Can you work these out from the drawing? Everything is in mm from the part's minimum corner. A direction names the side the tool comes from. Give positions to 0.01 mm unless a question says otherwise; leave off trailing zeros. Order: outer loops, then holes, each group sorted by start corner. A loop starts at its lowest first (then second) coordinate and runs counter-clockwise, first axis right, second up. Notation, with made-up numbers: (24.5, 53) -> (79.5, 53) arc R32 cw to (79.5, 83) -> close; hole circle Ø6 at (-30.75, -40). An arc over 180 degrees is marked (long way). One line per item, written item: value.
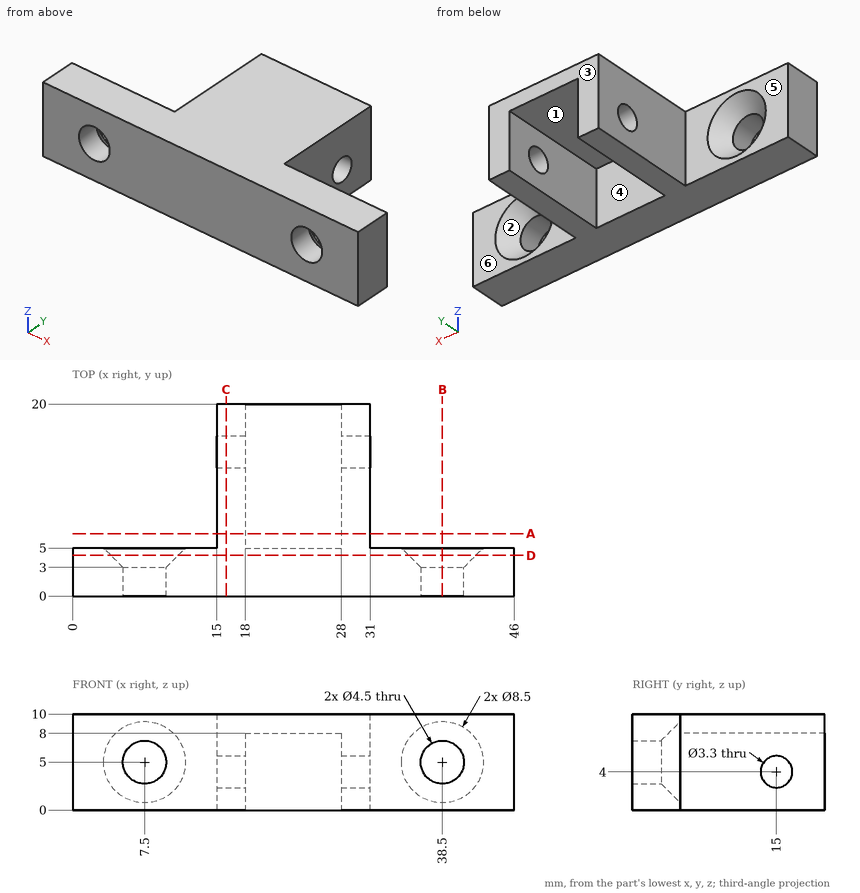
1) Suppose I cut it at C-C, the plane x = 16. Write out the boundary of the cut face in (y, z).
Answer below:
outline: (0, 0) -> (20, 0) -> (20, 10) -> (0, 10) -> close; hole circle Ø3.3 at (15, 4)
2) We'd pull the mould along Z, two halves only. Please class the marked faces 1, 2 and 3: +Z half, -Z half, draft (parallel to the pull), parting line (faces both ways), or undercut.
Answer below:
face 1: -Z half
face 2: undercut
face 3: draft
3) Suppose I cut it at B-B, the plane x = 38.5. Write out the boundary of the cut face in (y, z), then the cut area to 3 significant figures.
Answer below:
outline: (0, 0) -> (5, 0) -> (5, 0.75) -> (3, 2.75) -> (0, 2.75) -> close; (0, 7.25) -> (3, 7.25) -> (5, 9.25) -> (5, 10) -> (0, 10) -> close
area: 23.5 mm2
4) Suppose I cut it at D-D, the plane y = 4.25. Write out the boundary of the cut face in (x, z), then the cut area to 3 significant figures.
Answer below:
outline: (0, 0) -> (46, 0) -> (46, 10) -> (0, 10) -> close; hole circle Ø7 at (7.5, 5); hole circle Ø7 at (38.5, 5)
area: 383 mm2
5) For the marked faces 4, 5 and 6, which set-ups out of +Z, -Z, +X, -X, +Y, -Y let a thin tool reach every point of the face, with its end or its side?
Answer below:
face 4: -Z, +Y
face 5: +Z, -Z, -X, +Y
face 6: +Z, -Z, +X, +Y
6) If I drill on line 1 along X through (y, z) = (9.5, 1.5); line 2 along Z through (x, y) = (16.8, 15); line 3 along Y through (x, z) = (39, 0.75), over which ranges is the centre line in solid material (lowest first)?
Answer below:
line 1: x = 15 to 18, 28 to 31
line 2: z = 0 to 2.35, 5.65 to 10
line 3: y = 0 to 5
7) For P1, Ø4, axis at x = 24, z = 4.5, coming from the +Y side; P2, Ø3, axis at x = 9.5, z = 6, coming from the +Y side; P3, Ø3, axis at y = 12.5, z = 4.5, coming from the +X side, each with a flat end and sliding along its axis, tell me the tip position at first contact or that it passes through.
Answer below:
P1: stops at y = 5
P2: stops at y = 4.49
P3: stops at x = 31
8) Suppose I cut it at A-A, the plane y = 6.5. Write out the boundary of the cut face in (x, z).
Answer below:
outline: (15, 0) -> (18, 0) -> (18, 8) -> (28, 8) -> (28, 0) -> (31, 0) -> (31, 10) -> (15, 10) -> close
